Here's the drawing with two shaded views (mm, measured from the low corner). I have some questions. Coordinates: 2 decimals unless noted, no trailing zeros. Loops run counter-clockwise (first coordinate to the right, second up) from the corner with the lowest first, then second, coordinate; pieces in that order, holes last.
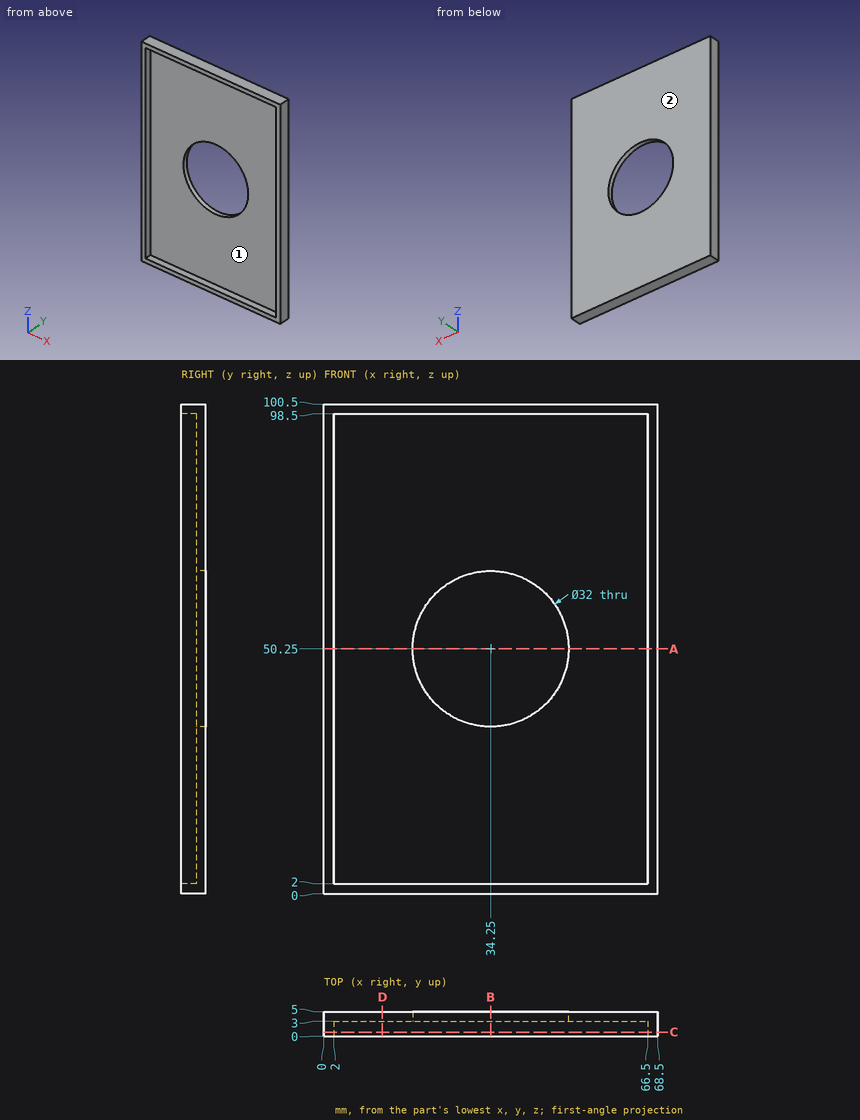
(1) I want a section at D-D on x = 12. Write out the boundary of the cut face in (y, z).
Check values:
outline: (0, 0) - (5, 0) - (5, 100.5) - (0, 100.5) - (0, 98.5) - (3, 98.5) - (3, 2) - (0, 2) - close
(2) I want a section at C-C on y = 0.8. Write out the boundary of the cut face in (x, z).
Check values:
outline: (0, 0) - (68.5, 0) - (68.5, 100.5) - (0, 100.5) - close; hole (2, 2) - (66.5, 2) - (66.5, 98.5) - (2, 98.5) - close
(3) I want a section at B-B on x = 34.25. Write out the boundary of the cut face in (y, z).
Check values:
outline: (0, 0) - (5, 0) - (5, 34.25) - (3, 34.25) - (3, 2) - (0, 2) - close; (0, 98.5) - (3, 98.5) - (3, 66.25) - (5, 66.25) - (5, 100.5) - (0, 100.5) - close
(4) If I drill on probe 1 along X at (y, z) = (2.05, 35.5); probe 2 along Z at (x, y) = (6.5, 1.25); probe 3 along Z at (x, y) = (34.25, 4.55), over which ranges is the centre line in solid material (lowest first)?
Check values:
probe 1: x = 0 to 2, 66.5 to 68.5
probe 2: z = 0 to 2, 98.5 to 100.5
probe 3: z = 0 to 34.25, 66.25 to 100.5
(5) I'm going to push a flat-ended pin straight in: pin 1 (8 mm diameter, centred on x = 54, z = 63, fed in from -Y). Where does the tip first touch, or does it pass through?
Check values:
pin 1: stops at y = 3
(6) If we mould it in two halves opening along Z, with no side actions, what happens to the marked faces 1 and 2? For each: released by +Z, released by -Z, zero draft, split by the parting line, or undercut.
Check values:
face 1: undercut
face 2: zero draft
(7) I want a section at A-A on z = 50.25. Write out the boundary of the cut face in (x, y), then the cut area to 3 significant figures.
Check values:
outline: (0, 0) - (2, 0) - (2, 3) - (18.25, 3) - (18.25, 5) - (0, 5) - close; (50.25, 3) - (66.5, 3) - (66.5, 0) - (68.5, 0) - (68.5, 5) - (50.25, 5) - close
area: 85.0 mm2
